Can you work these out from the model? Positions are in its coordinate system, mm. A direction names the side the tool comes from. Give positions to 0.01 mm unless a question says otherwise; leave off trailing zeros. Order: outer loops, then holes, each group sorted by start corner. A loop starts at its lowest first (then second) coordinate and runs counter-clockwise, first axis right, second up. Notation, with made-up numbers: M -17.5,-27 L -8.5,-27 A23 cw -8.5,5 Z; hole C 33,52 d11. An arc over 180 degrees is marked long. Answer as a JSON object with one key per item and string values.
```python
from build123d import *

# Parameters (mm, degrees)
EXTRUDE_1_DEPTH     = 3
SKETCH_3_R          = 1.75
CUT_EXTRUDE_1_DEPTH = 10


with BuildPart() as part:
    # Эскиз1 → Бобышка-Вытянуть1 (new body)
    with BuildSketch(Plane(origin=(0, 0, 0), x_dir=(1, 0, 0), z_dir=(0, 1, 0))):
        with BuildLine():
            Line((1.303877519, 4.981364115), (2.425804873, 6.229215237))
            ThreePointArc((2.425804873, 6.229215237), (4.642715437, 9.781674692), (7.001370076, 6.321702305))
            Line((7.001370076, 6.321702305), (10.562616141, 2.623485237))
            Line((10.562616141, 2.623485237), (10.919592499, 2.967240249))
            Line((10.919592499, 2.967240249), (10.919592499, 4.300759927))
            Line((10.919592499, 4.300759927), (11.728649514, 4.300759927))
            Line((11.728649514, 4.300759927), (11.728649514, 3.252739503))
            Line((11.728649514, 3.252739503), (11.728649514, 1.930836158))
            Line((11.728649514, 1.930836158), (10.117222577, 0.3790917))
            Line((10.117222577, 0.3790917), (7.157448349, 3.452703399))
            ThreePointArc((7.157448349, 3.452703399), (4.707383461, 4.814595243), (2.287238645, 3.400216789))
            Line((2.287238645, 3.400216789), (1.842702366, 2.922219258))
            Line((1.842702366, 2.922219258), (-0.547473895, 2.922219258))
            Line((-0.547473895, 2.922219258), (-4.731054927, 2.922219258))
            Line((-4.731054927, 2.922219258), (-4.731054927, 4.981364115))
            Line((-4.731054927, 4.981364115), (1.303877519, 4.981364115))
        make_face()
    extrude(amount=EXTRUDE_1_DEPTH)

    # Эскиз3 → Вырез-Вытянуть1 (cut)
    with BuildSketch(Plane(origin=(0, 3, 0), x_dir=(1, 0, 0), z_dir=(0, 1, 0))):
        with Locations(Location((4.693238255, 7.282185255, 0), (0, 0, 270))):
            Circle(SKETCH_3_R)
    extrude(amount=-CUT_EXTRUDE_1_DEPTH, mode=Mode.SUBTRACT)


solid = part.part
```
1) I want a section at D-D on y = 1.1. Write out the boundary of the cut face in (x, z), and give its area (3 significant figures).
Results found:
{"outline": "M -4.73,-4.98 L 1.3,-4.98 L 2.43,-6.23 A2.5 ccw long 7,-6.32 L 10.56,-2.62 L 10.92,-2.97 L 10.92,-4.3 L 11.73,-4.3 L 11.73,-1.93 L 10.12,-0.38 L 7.16,-3.45 A2.83 cw 2.29,-3.4 L 1.84,-2.92 L -4.73,-2.92 Z; hole C 4.69,-7.28 d3.5", "area": "40.9 mm²"}
2) I want a section at C-C on x = 5. Write out the boundary of the cut face in (y, z).
Results found:
{"outline": "M 0,-9.76 L 3,-9.76 L 3,-9.01 L 0,-9.01 Z; M 0,-5.56 L 3,-5.56 L 3,-4.8 L 0,-4.8 Z"}
3) I need wall thicknesses on L1, parallel to Z at x = 4.75, y = 0.8; L2, parallel to X at y = 0.4, z = -3.75; L3, parallel to Z at x = -2.5, y = 2.25. Which ranges of each line are inside material? Lowest first, please.
Results found:
{"L1": "z = -9.78 to -9.03, -5.53 to -4.81", "L2": "x = -4.73 to 2.53, 6.95 to 9.48, 10.92 to 11.73", "L3": "z = -4.98 to -2.92"}
4) For faces 4 (the face through (-2, 1, -4.981)), 5 (the face through (1.86, 1.48, -5.6)), 6 (the face through (11.3, 1.5, -4.301)), 7 (the face through (-1, 1, -2.922)), which set-ups out of +Z, -Z, +X, -X, +Y, -Y let a thin tool reach every point of the face, with its end or its side?
Results found:
{"face 4": "-Z, -X, +Y, -Y", "face 5": "-X, +Y, -Y", "face 6": "-Z, +X, +Y, -Y", "face 7": "+Z, -X, +Y, -Y"}
5) I want a section at B-B on z = -6.75. Write out the boundary of the cut face in (x, y).
Results found:
{"outline": "M 2.25,0 L 3.03,0 L 3.03,3 L 2.25,3 Z; M 6.36,0 L 7.14,0 L 7.14,3 L 6.36,3 Z"}
6) Thinking about a two-plate mould opening in X: for faces 1 (the face through (10.934, 1.479, -1.166)), 2 (the face through (8.757, 1.479, -4.498)), 3 (the face through (4, 3, -5)), which applies, pulls with the +X half, pulls with the -X half, needs draft (parallel to the pull), parting line crosses it, or undercut?
Results found:
{"face 1": "pulls with the +X half", "face 2": "undercut", "face 3": "needs draft"}
7) I'm going to push flat-ended pins straight in: pin 1 Ø0.9 at (x, y) = (-0.5, 1.5) entering from -Z; pin 2 Ø1.5 at (x, y) = (8, 2) entering from +Z. Where does each tip first touch, or does it pass through?
Results found:
{"pin 1": "stops at z = -4.98", "pin 2": "stops at z = -1.8"}
8) I want a section at A-A on z = -4. Write out the boundary of the cut face in (x, y).
Results found:
{"outline": "M -4.73,0 L 2.75,0 L 2.75,3 L -4.73,3 Z; M 6.72,0 L 9.24,0 L 9.24,3 L 6.72,3 Z; M 10.92,0 L 11.73,0 L 11.73,3 L 10.92,3 Z"}
